Print and shaded views of the part. All mm, measured from the part's lowest x, y and z. A direction names the side the tool comes from. Round coordinates to 2 decimals unless told otherwise and drop trailing zeros. Order: outer loops, then holes, each group sorted by start corner. A loop starts at its lowest first (then second) coordinate and runs counter-clockwise, first axis right, second up. Notation, with made-up numbers: (46.5, 45) - (105.5, 45) arc R22 cw to (105.5, 61) - close; hole circle Ø8 at (57.25, -19.5). An arc over 180 degrees is marked (long way). Write item = value, one per line.
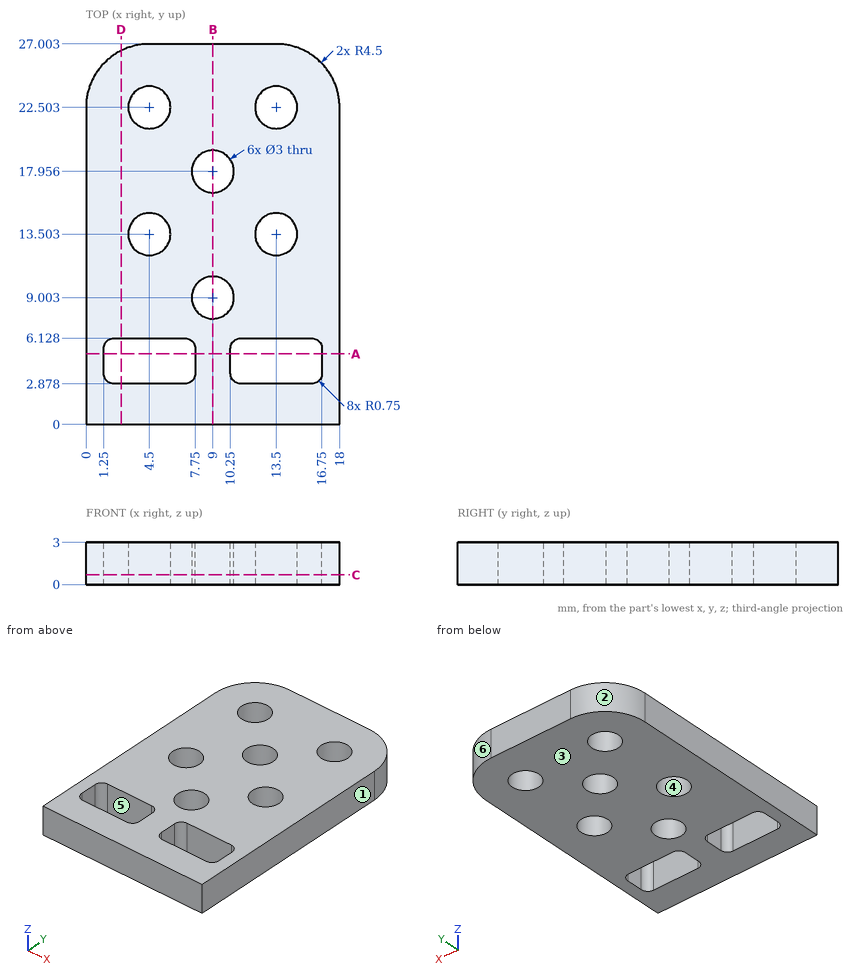
(1) Probe line 1 along X through (y, z) = (5, 0.5); line 2 along Y through (x, z) = (4.5, 0.9); line 3 along X through (y, z) = (22.5, 1.45). List the from-to ranges inside material, lowest first.
Solved:
line_1 = 0 to 1.25, 7.75 to 10.25, 16.75 to 18
line_2 = 0 to 2.88, 6.13 to 12, 15 to 21, 24 to 27
line_3 = 0 to 3, 6 to 12, 15 to 18
(2) Drop a flat-ended pin along its axis: pin 1 (1.8 mm diameter, centred on x = 13.5, y = 13.5, fed in from -Z). Give the stop position or say it passes through.
Solved:
pin_1 = through
(3) Band-saw the part on C-C on z = 0.7. Count the separate pieces of the cut face and the enclosed holes in it, plus the area to 3 significant figures.
Solved:
separate_pieces = 1
enclosed_holes = 8
area = 394 mm²
(4) Band-saw the part on B-B on x = 9. List the corners of the cut face in (y, z), plus the area to 3 significant figures.
Solved:
outline = (0, 0) - (7.5, 0) - (7.5, 3) - (0, 3) - close; (10.5, 0) - (16.46, 0) - (16.46, 3) - (10.5, 3) - close; (19.46, 0) - (27, 0) - (27, 3) - (19.46, 3) - close
area = 63.0 mm²
(5) Tool access for the marked faces 5 and 6: list every direction of +Z, -Z, +X, -X, +Y, -Y with a clear straight run to the whole face (end or side of a thin tool).
Solved:
face_5 = +Z, -Z
face_6 = +Z, -Z, +X, +Y
(6) Band-saw the part on D-D on x = 2.5. List the corners of the cut face in (y, z).
Solved:
outline = (0, 0) - (2.88, 0) - (2.88, 3) - (0, 3) - close; (6.13, 0) - (26.53, 0) - (26.53, 3) - (6.13, 3) - close
(7) Pull direction X, two halves, no side cores. Call the marked faces 1, 2, 3 and 4: released by +X, released by -X, zero draft, split by the parting line, or undercut.
Solved:
face_1 = released by +X
face_2 = released by -X
face_3 = zero draft
face_4 = undercut
(8) Band-saw the part on A-A on y = 5. List the corners of the cut face in (x, z), plus the area to 3 significant figures.
Solved:
outline = (0, 0) - (1.25, 0) - (1.25, 3) - (0, 3) - close; (7.75, 0) - (10.25, 0) - (10.25, 3) - (7.75, 3) - close; (16.75, 0) - (18, 0) - (18, 3) - (16.75, 3) - close
area = 15.0 mm²
